Geometry: see drawing. Coordinates: mm, zero at the bounding-box minimum. Round coordinates to 2 decimals unless told otherwise and drop trailing zeros. Write each loop counter-clockwise with the first axis right and the second up, starting at its lowest first coordinate (ties: lowest second). Pieces come first, ordered by that corner, then holes. Notation, with made-up numbers: (88.5, 19) -> (133.5, 19) arc R19 ccw to (133.5, 50) -> close; hole circle Ø1 at (81, 52). An arc over 180 degrees is marked (long way). Write item = value, one per line.
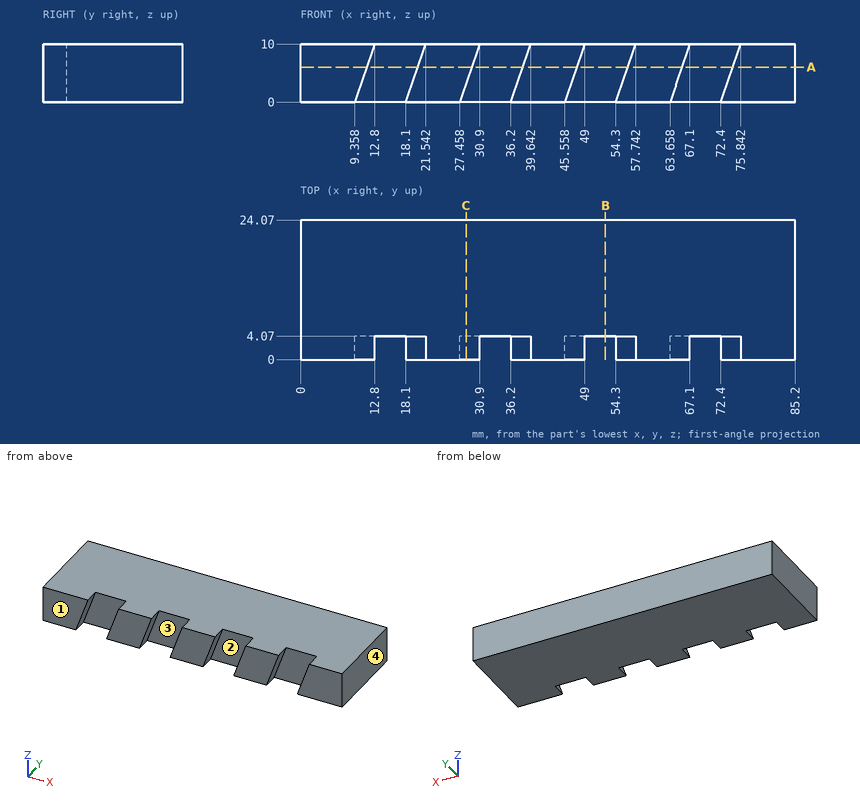
1) Cut plane A-A (z = 6). Return the cut outline in (x, y) (1 decimal).
Solutions:
outline = (0, 0) -> (11.4, 0) -> (11.4, 4.1) -> (20.2, 4.1) -> (20.2, 0) -> (29.5, 0) -> (29.5, 4.1) -> (38.3, 4.1) -> (38.3, 0) -> (47.6, 0) -> (47.6, 4.1) -> (56.4, 4.1) -> (56.4, 0) -> (65.7, 0) -> (65.7, 4.1) -> (74.5, 4.1) -> (74.5, 0) -> (85.2, 0) -> (85.2, 24.1) -> (0, 24.1) -> close
2) Cut plane B-B (x = 52.5). Return the cut outline in (y, z).
Solutions:
outline = (4.07, 0) -> (24.07, 0) -> (24.07, 10) -> (4.07, 10) -> close
3) Line query: L1, parallel to Y at x = 70, z = 8.75. Output: solid intervals per line, ascending. Write a range as from..to.
Solutions:
L1 = 4.07..24.07
4) First-contact query: P1, Ø6, axis at y = 13, z = 6.5, coming from the -X side; P2, Ø5, axis at x = 34.5, z = 7, coming from the -Y side. Flat tips, straight axial feed; report the tip coordinate or a pass-through.
Solutions:
P1 = 0
P2 = 4.07
5) Draft query along X for the marked faces 1, 2, 3 and 4. Return one class per face: +X half, -X half, draft (parallel to the pull), parting line (faces both ways), or undercut.
Solutions:
face_1 = draft
face_2 = undercut
face_3 = undercut
face_4 = +X half
6) Cut plane C-C (x = 28.5). Return the cut outline in (y, z), and give its area (3 significant figures).
Solutions:
outline = (0, 3.03) -> (4.07, 3.03) -> (4.07, 0) -> (24.07, 0) -> (24.07, 10) -> (0, 10) -> close
area = 228 mm^2
